Can you work these out from the model? Positions are in its coordinate system, mm. A direction names the side the tool comes from. Coordinates: 2 decimals unless noted, no trailing zeros. Order: outer loops, then holes, each group sorted by start corner. A loop starts at its lowest first (then second) coordinate and runs counter-clockwise, first axis right, second up. Notation, with made-up numbers: (56.25, 77.25) -> (77.25, 77.25) arc R10 cw to (77.25, 81.25) -> close; hole circle Ø1 at (62, -14). An arc over 180 degrees is marked (long way). Return JSON: item names as keys, results as strings. Group by question number.
1) If we section it at B-B, the plane x = -10: Please give me the cut outline in (y, z).
2) If we section it at A-A, the plane y = 0: Please give me the cut outline in (x, z), then the cut area to 4 significant figures.
3) If I drill on probe 1 along Z at (x, y) = (-3.75, 0.45); probe 2 along Z at (x, y) = (-0.5, -0.2); probe 3 along X at (y, z) = (0.75, -0.5), over which ranges is the centre line in solid material (lowest first)? Write a range as from..to.
4) For pin 1 (1.1 mm diameter, centred on x = -1.5, y = -1.5, fed in from +Z); pin 2 (1 mm diameter, centred on x = -1, y = 0, fed in from -Z), each with a flat end and sliding along its axis, tell me the tip position at first contact or that it passes through.
5) For faces 1 (the cylindrical face through (-10.04, -1.25, -2.46)), 2 (the cylindrical face through (0.04, -1.25, 6.09)), 3 (the flat face through (-5, 1, 2)), which set-ups out of +Z, -Z, +X, -X, +Y, -Y let a thin tool reach every point of the face, with its end or its side?
6) If we section it at C-C, the plane z = -1: Please give me the cut outline in (x, y), then the cut area to 3 significant figures.
7) If we section it at D-D, the plane y = -0.75: Please give me the cut outline in (x, z), then the cut area to 4 significant figures.
Autodesk Inventor part; units mm, degrees
ref_plane "YZ Plane" through (0, 0, 0) normal (1, 0, 0) x (0, 1, 0)
ref_plane "XZ Plane" through (0, 0, 0) normal (0, 1, 0) x (-1, 0, 0)
ref_plane "XY Plane" through (0, 0, 0) normal (0, 0, 1) x (1, 0, 0)
sketch "Sketch1" plane through (0, 0, 0) normal (0, 0, 1) x (1, 0, 0)
  circle A0 centre (0, 0) radius 1.25
  circle A1 centre (0, 0) radius 2.75
  line L0 (-1.75, 2.75) -> (1.75, 2.75)
  line L1 (2.75, 1.75) -> (2.75, -1.75)
  line L2 (1.75, -2.75) -> (-1.75, -2.75)
  line L3 (-2.75, -1.75) -> (-2.75, 1.75)
  arc A2 (-1.75, 2.75) -> (-2.75, 1.75) centre (-1.75, 1.75) ccw
  arc A3 (2.75, 1.75) -> (1.75, 2.75) centre (1.75, 1.75) ccw
  arc A4 (1.75, -2.75) -> (2.75, -1.75) centre (1.75, -1.75) ccw
  arc A5 (-2.75, -1.75) -> (-1.75, -2.75) centre (-1.75, -1.75) ccw
  line L4 (-2.75, 1) -> (2.75, 1)
  line L5 (0, 2.75) -> (-11.75, 2.75)
  line L6 (-12.75, 1.75) -> (-12.75, -1.75)
  line L7 (-11.75, -2.75) -> (0, -2.75)
  line L8 (0, -2.75) -> (0, 2.75)
  circle A6 centre (-10, 0) radius 2.75
  circle A7 centre (-10, 0) radius 1.25
  line L9 (-2.75, 1) -> (-12.75, 1)
  arc A8 (-11.75, 2.75) -> (-12.75, 1.75) centre (-11.75, 1.75) ccw
  arc A9 (-12.75, -1.75) -> (-11.75, -2.75) centre (-11.75, -1.75) ccw
  point P0 (-2.75, 0)
  point P1 (0, -2.75)
  point P2 (0.75, 1)
  point P3 (-0.75, 1)
  point P4 (0, 0)
  point P5 (-9.25, 1)
  point P6 (-10.75, 1)
  dimension "d0" = 2.5
  dimension "d1" = 5.5
  dimension "d2" = 1
  dimension "d3" = 1
  dimension "d4" = 1
  dimension "d11" = 1
  dimension "d12" = 2.5
  dimension "d13" = 10
  dimension "d14" = 1
extrude "Extrusion1" add sketch "Sketch1" along normal blind 7.1 contours A0 L8 L4 | A0 L4 L8 picked at (0.0927, -0.4896) picked at (-0.103, -0.4871)
extrude "Extrusion2" add sketch "Sketch1" along normal blind 5.1 contours A0 L8 L4 | A0 L4 A1 L8 | L8 A1 L4 A0 | A0 L4 L8 | L4 L1 A1 | L2 A5 L3 A1 | A1 L1 A4 L2 | A1 L3 L4 | L3 A5 L7 A6 L9 | L7 A9 L6 A6 | A6 L9 A7 | L6 L9 A6 | A7 L9 picked at (0.0927, -0.4896) picked at (2.2166, -0.2967) picked at (-0.204, -2.227) picked at (-0.103, -0.4871) picked at (-7.773, -0.204) picked at (-10.4044, -0.1231)
extrude "Extrusion3" add sketch "Sketch1" against normal blind 5 contours A7 L9 picked at (-10.4044, -0.1231)
equation "\"d12\" = d0"
properties part number "rpi_base_front_3DPrint"
Result sheet:
{
 "1": {"outline": "(-2.75, 0) -> (-1.25, 0) -> (-1.25, -5) -> (1, -5) -> (1, 5.1) -> (-2.75, 5.1) -> close"},
 "2": {"outline": "(-12.75, 0) -> (-11.25, 0) -> (-11.25, -5) -> (-8.75, -5) -> (-8.75, 0) -> (2.75, 0) -> (2.75, 5.1) -> (1.25, 5.1) -> (1.25, 7.1) -> (-1.25, 7.1) -> (-1.25, 5.1) -> (-12.75, 5.1) -> close", "area": "96.55 mm2"},
 "3": {"probe 1": "z = 0..5.1", "probe 2": "z = 0..7.1", "probe 3": "x = -11..-9"},
 "4": {"pin 1": "stops at z = 5.1", "pin 2": "stops at z = 0"},
 "5": {"face 1": "-Z", "face 2": "+Z", "face 3": "+Z, -Z, +X, -X, +Y"},
 "6": {"outline": "(-10.75, 1) arc R1.25 ccw (long way) to (-9.25, 1) -> close", "area": "4.65 mm2"},
 "7": {"outline": "(-12.75, 0) -> (-11, 0) -> (-11, -5) -> (-9, -5) -> (-9, 0) -> (2.75, 0) -> (2.75, 5.1) -> (1, 5.1) -> (1, 7.1) -> (-1, 7.1) -> (-1, 5.1) -> (-12.75, 5.1) -> close", "area": "93.05 mm2"}
}
